Check sheet for the modelled part. Datum: model origin and axes. Units: mm. A direction names the side the tool comes from. Round coordinates to 2 decimals unless told otherwise and drop trailing zeros. Write each loop counter-clockwise with the first axis right and the second up, starting at its lowest first coordinate (ties: lowest second). Pieces come first, ordered by that corner, then holes.
Item 1: Material ranges on line 1 along Z through (x, y) = (16.5, 11); line 2 along X through (y, z) = (9.5, -38); line 3 along X through (y, z) = (10.5, -33), recorded low to high.
Item 2: Section check B-B, the plane y = 8. State how many separate pieces and enclosed holes the cut face has, plus the area to 3 significant figures.
Item 3: Release check for a two-part mould opening along X. For faces 4 (the flat face through (3.504, 6, -24)), 5 (the flat face through (9, 11.938, -47)), 6 (the flat face through (15.061, 6, -11)), 7 (the flat face through (7.695, 6, -6)) record: pulls with the +X half, pulls with the -X half, needs draft (parallel to the pull), parting line crosses it, or undercut.
Item 4: Set-up check for faces 1 (the flat face through (1, 6, -8.712)), 2 (the flat face through (16.077, 6, -44)), 3 (the flat face through (20.395, 6, -15)): record each of +Z, -Z, +X, -X, +Y, -Y from which the full face is reachable in a straight line by a thin tool's end or side.
Item 5: Section check A-A, the plane z = -33. Record the cut outline in (x, y).
Item 6: Depth check by flat-ended pin: pin 1 (1 mm diameter, centred on y = 7.5, z = -2, fed in from -X); pin 2 (4.5 mm diameter, centred on y = 6, z = -10.5, fed in from -X); pin 3 (3.5 mm diameter, centred on x = 0.5, y = 3.5, fed in from -Z). Enter the tip coordinate at first touch or a pass-through.
from build123d import *

# Parameters (mm, degrees)
F0_W      = 25.4
F0_H      = 30.48
F1_DEPTH  = 1.016
F2_W      = 1.016
F2_H      = 10.16
F2_H_2    = 9.144
F2_W_2    = 8.382
F2_H_3    = 1.016
F3_DEPTH  = 1.017
F4_W      = 25.4
F4_H      = 30.48
F5_DEPTH  = 1.016
F6_W      = 1.016
F6_H      = 9.144
F6_W_2    = 8.382
F6_H_2    = 1.016
F6_H_3    = 10.16
F7_DEPTH  = 1.017
F8_W      = 5.334
F8_H      = 13.462
F8_W_2    = 3.302
F8_H_2    = 11.43
F8_H_3    = 10.414
F8_W_3    = 11.43
F8_H_4    = 5.334
F8_W_4    = 9.652
F8_H_5    = 3.302
F8_W_5    = 0.127
F8_H_6    = 0.0508
F9_DEPTH  = 12.954
F10_W     = 1.524
F10_H     = 60.96
F11_DEPTH = 25.4


with BuildPart() as f1:
    # F0 (on Front) → F1 (new body)
    with BuildSketch(Plane.XZ):
        with Locations((9.3459782816, -10.94705052)):
            Rectangle(F0_W, F0_H)
    extrude(amount=F1_DEPTH)

    # F2 (on Front) → F3 (cut, through all)
    with BuildSketch(Plane.XZ):
        with Locations((9.3459782816, -5.48605052)):
            Rectangle(F2_W, F2_H)
        with Locations((0.9639782816, -14.93485052)):
            Rectangle(F2_W, F2_H_2)
        with Locations((17.7279782816, -14.93485052)):
            Rectangle(F2_W, F2_H_2)
        with Locations((9.3459782816, -15.64605052)):
            Rectangle(F2_W_2, F2_H_3)
        with Locations((9.3459782816, -23.77405052)):
            Rectangle(F2_W_2, F2_H_3)
    extrude(amount=F3_DEPTH, mode=Mode.SUBTRACT)

    # F4 (on face) → F5 (join)
    with BuildSketch(Plane.XZ.offset(1.016)):
        with Locations((9.3459782816, -41.42705052)):
            Rectangle(F4_W, F4_H)
    extrude(amount=-F5_DEPTH)

    # F6 (on face) → F7 (cut, through all)
    with BuildSketch(Plane.XZ.offset(1.016)):
        with Locations((0.9639782816, -14.93485052)):
            Rectangle(F6_W, F6_H)
        with Locations((9.3459782816, -15.64605052)):
            Rectangle(F6_W_2, F6_H_2)
        with Locations((9.3459782816, -5.48605052)):
            Rectangle(F6_W, F6_H_3)
        with Locations((17.7279782816, -14.93485052)):
            Rectangle(F6_W, F6_H)
        with Locations((9.3459782816, -23.77405052)):
            Rectangle(F6_W_2, F6_H_2)
        with Locations((9.3459782816, -34.69605052)):
            Rectangle(F6_W, F6_H_3)
        with Locations((17.7279782816, -44.14485052)):
            Rectangle(F6_W, F6_H)
        with Locations((9.3459782816, -44.85605052)):
            Rectangle(F6_W_2, F6_H_2)
        with Locations((9.3459782816, -52.98405052)):
            Rectangle(F6_W_2, F6_H_2)
        with Locations((0.9639782816, -44.14485052)):
            Rectangle(F6_W, F6_H)
    extrude(amount=-F7_DEPTH, mode=Mode.SUBTRACT)

    # F8 (on face) → F9 (join)
    with BuildSketch(Plane.XZ.offset(1.016)):
        with Locations((9.3459782816, -5.48605052)):
            Rectangle(F8_W, F8_H)
        with Locations((9.3459782816, -5.48605052)):
            Rectangle(F8_W_2, F8_H_2, mode=Mode.SUBTRACT)
        Polygon((3.6309782816, -12.97905052), (3.6309782816, -8.71185052), (-1.7030217184, -8.71185052), (-1.7030217184, -21.15785052), (3.5039782816, -21.15785052), (3.5039782816, -21.10705052), (3.6309782816, -21.10705052), (3.6309782816, -18.31305052), (3.5039782816, -18.31305052), (3.5039782816, -12.97905052), align=None)
        with Locations((0.9639782816, -14.93485052)):
            Rectangle(F8_W_2, F8_H_3, mode=Mode.SUBTRACT)
        with Locations((9.3459782816, -15.64605052)):
            Rectangle(F8_W_3, F8_H_4)
        with Locations((9.3459782816, -15.64605052)):
            Rectangle(F8_W_4, F8_H_5, mode=Mode.SUBTRACT)
        with Locations((3.5674782816, -15.64605052)):
            Rectangle(F8_W_5, F8_H_4)
        with Locations((15.1244782816, -15.64605052)):
            Rectangle(F8_W_5, F8_H_4)
        Polygon((15.0609782816, -8.71185052), (15.0609782816, -12.97905052), (15.1879782816, -12.97905052), (15.1879782816, -18.31305052), (15.0609782816, -18.31305052), (15.0609782816, -21.10705052), (15.1879782816, -21.10705052), (15.1879782816, -21.15785052), (20.3949782816, -21.15785052), (20.3949782816, -8.71185052), align=None)
        with Locations((17.7279782816, -14.93485052)):
            Rectangle(F8_W_2, F8_H_3, mode=Mode.SUBTRACT)
        with Locations((3.5674782816, -21.13245052)):
            Rectangle(F8_W_5, F8_H_6)
        Polygon((3.6309782816, -21.15785052), (3.5039782816, -21.15785052), (3.5039782816, -26.44105052), (15.1879782816, -26.44105052), (15.1879782816, -21.15785052), (15.0609782816, -21.15785052), (15.0609782816, -21.10705052), (3.6309782816, -21.10705052), align=None)
        with Locations((9.3459782816, -23.77405052)):
            Rectangle(F8_W_4, F8_H_5, mode=Mode.SUBTRACT)
        with Locations((15.1244782816, -21.13245052)):
            Rectangle(F8_W_5, F8_H_6)
        with Locations((9.3459782816, -34.69605052)):
            Rectangle(F8_W, F8_H)
        with Locations((9.3459782816, -34.69605052)):
            Rectangle(F8_W_2, F8_H_2, mode=Mode.SUBTRACT)
        Polygon((20.3949782816, -37.92185052), (15.0609782816, -37.92185052), (15.0609782816, -42.18905052), (15.1879782816, -42.18905052), (15.1879782816, -47.52305052), (15.0609782816, -47.52305052), (15.0609782816, -50.31705052), (15.1879782816, -50.31705052), (15.1879782816, -50.36785052), (20.3949782816, -50.36785052), align=None)
        with Locations((17.7279782816, -44.14485052)):
            Rectangle(F8_W_2, F8_H_3, mode=Mode.SUBTRACT)
        with Locations((15.1244782816, -44.85605052)):
            Rectangle(F8_W_5, F8_H_4)
        with Locations((9.3459782816, -44.85605052)):
            Rectangle(F8_W_3, F8_H_4)
        with Locations((9.3459782816, -44.85605052)):
            Rectangle(F8_W_4, F8_H_5, mode=Mode.SUBTRACT)
        with Locations((3.5674782816, -44.85605052)):
            Rectangle(F8_W_5, F8_H_4)
        Polygon((3.5039782816, -42.18905052), (3.6309782816, -42.18905052), (3.6309782816, -37.92185052), (-1.7030217184, -37.92185052), (-1.7030217184, -50.36785052), (3.5039782816, -50.36785052), (3.5039782816, -50.31705052), (3.6309782816, -50.31705052), (3.6309782816, -47.52305052), (3.5039782816, -47.52305052), align=None)
        with Locations((0.9639782816, -44.14485052)):
            Rectangle(F8_W_2, F8_H_3, mode=Mode.SUBTRACT)
        with Locations((15.1244782816, -50.34245052)):
            Rectangle(F8_W_5, F8_H_6)
        Polygon((15.0609782816, -50.36785052), (15.0609782816, -50.31705052), (3.6309782816, -50.31705052), (3.6309782816, -50.36785052), (3.5039782816, -50.36785052), (3.5039782816, -55.65105052), (15.1879782816, -55.65105052), (15.1879782816, -50.36785052), align=None)
        with Locations((9.3459782816, -52.98405052)):
            Rectangle(F8_W_4, F8_H_5, mode=Mode.SUBTRACT)
        with Locations((3.5674782816, -50.34245052)):
            Rectangle(F8_W_5, F8_H_6)
    extrude(amount=-F9_DEPTH)

    # F10 (on face) → F11 (cut)
    with BuildSketch(Plane.XZ.offset(1.016)):
        with Locations((-2.5920217184, -26.18705052)):
            Rectangle(F10_W, F10_H)
    extrude(amount=-F11_DEPTH, mode=Mode.SUBTRACT)


solid = f1.part
Values found:
1. line 1: z = -50.37 to -49.35, -38.94 to -37.92, -21.16 to -20.14, -9.73 to -8.71
1. line 2: x = -1.7 to 3.63, 6.68 to 7.69, 11 to 12.01, 15.06 to 20.39
1. line 3: x = 6.68 to 7.69, 11 to 12.01
2. separate pieces: 4
2. enclosed holes: 12
2. area: 315 mm2
3. face 4: pulls with the -X half
3. face 5: needs draft
3. face 6: undercut
3. face 7: undercut
4. face 1: +Z, -X, +Y
4. face 2: +Y
4. face 3: +Z, -Z, +X, +Y
5. outline: (-1.83, -1.02) - (8.84, -1.02) - (8.84, 0) - (7.69, 0) - (7.69, 11.94) - (6.68, 11.94) - (6.68, 0) - (-1.83, 0) - close; (9.85, -1.02) - (22.05, -1.02) - (22.05, 0) - (12.01, 0) - (12.01, 11.94) - (11, 11.94) - (11, 0) - (9.85, 0) - close
6. pin 1: stops at x = 6.68
6. pin 2: stops at x = -1.7
6. pin 3: stops at z = -50.37
